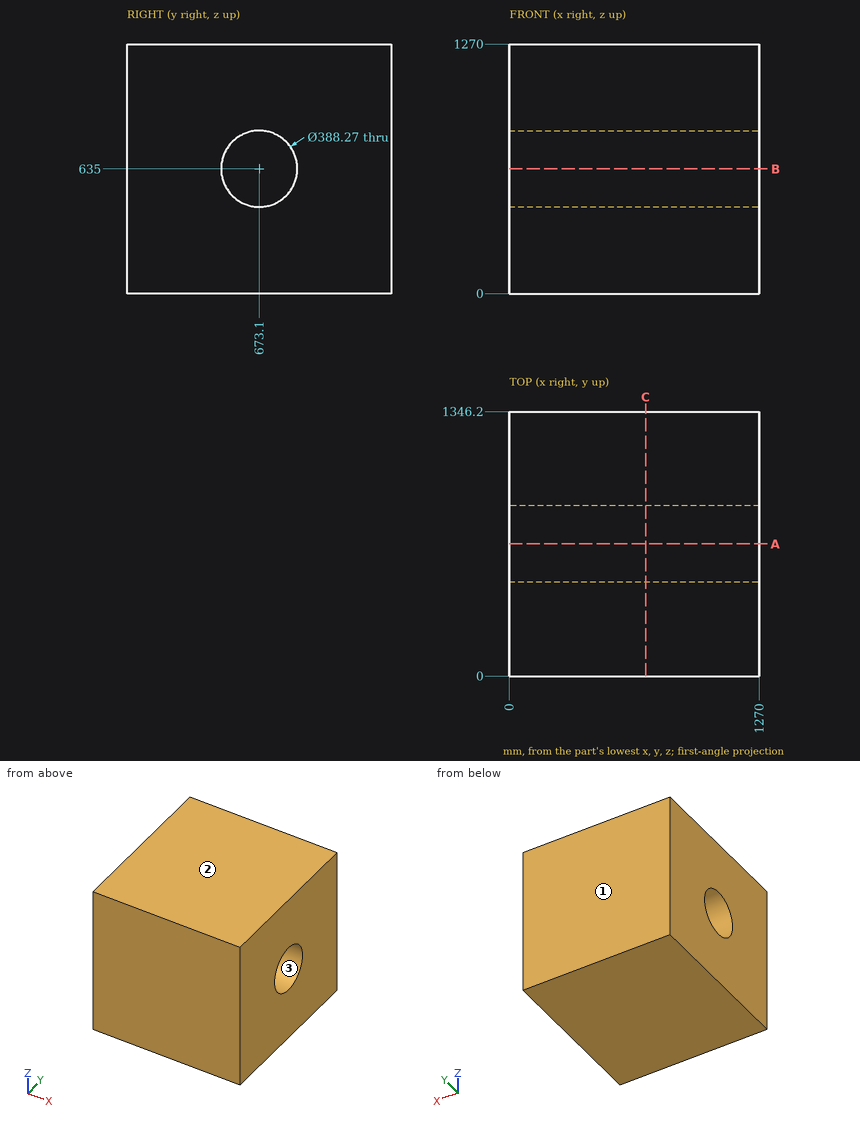
Study the drawing (mm; zero at the part's minimum x, y, z) and answer. Give positions to 0.01 mm unless a question says otherwise; leave off trailing zeros. Write each loop counter-clockwise with the first axis right and the second up, starting at its lowest first coordinate (ties: lowest second). Pieces come first, ordered by that corner, then holes. Notation, with made-up numbers: (57, 46.25) - (72, 46.25) arc R26 cw to (72, 79.25) - close; hole circle Ø10 at (16.25, 50). An arc over 180 degrees is marked (long way). One line per question, with ' | ' between items. Start each with the question number.
1. Straight lines are drawn through the part: line 1 (Z direction, x = 777, y = 673.1) (3 decimals); line 2 (Y direction, x = 839, z = 717.5); line 3 (Y direction, x = 549, z = 718). For each, find the intervals that lie inside material, in ascending order.
2. Section A-A, the plane y = 673.1 is taken. Determine the outline of the cut face in (x, z) (3 decimals).
3. Determine the mould class of the marked faces 1, 2 and 3 for opening direction Z: +Z half, -Z half, draft (parallel to the pull), parting line (faces both ways), or undercut.
4. Section C-C, the plane x = 693.5 is taken. Determine the outline of the cut face in (y, z) (3 decimals), then the cut area to 3 significant figures.
5. Section B-B, the plane z = 635 is taken. Determine the outline of the cut face in (x, y) (3 decimals).
Result:
1) line 1: z = 0 to 440.865, 829.135 to 1270 | line 2: y = 0 to 497.37, 848.83 to 1346.2 | line 3: y = 0 to 497.6, 848.6 to 1346.2
2) outline: (0, 0) - (1270, 0) - (1270, 440.865) - (0, 440.865) - close; (0, 829.135) - (1270, 829.135) - (1270, 1270) - (0, 1270) - close
3) face 1: draft | face 2: +Z half | face 3: undercut
4) outline: (0, 0) - (1346.2, 0) - (1346.2, 1270) - (0, 1270) - close; hole circle Ø388.27 at (673.1, 635) | area: 1,590,000 mm2
5) outline: (0, 0) - (1270, 0) - (1270, 478.965) - (0, 478.965) - close; (0, 867.235) - (1270, 867.235) - (1270, 1346.2) - (0, 1346.2) - close
